Read the model definition and answer for the solid it produces. Units are mm, in the model's axes. A direction names the side the tool comes from. Give positions to 0.01 mm unless a question says otherwise; leave off trailing zeros. Write each loop counter-clockwise with the first axis right and the second up, starting at its lowest first coordinate (ties: lowest second). Pieces come first, ordered by that corner, then holes. Notation, with made-up numbers: M -27.5,61.5 L -11.5,61.5 A25 cw -11.5,88.5 Z; hole C 56.5,35.25 d11. An arc over 180 degrees is marked long. Use a Markdown table: item, result. Add a question column.
Item 1: The mould has two halves that part along Y. Classify faces 1 (the flat face through (15, -1, 3)), 2 (the cylindrical face through (-12.2, -1.8, -2.4)), 3 (the cylindrical face through (-9.06, 5.16, -4.73)): pulls with the +Y half, pulls with the -Y half, needs draft (parallel to the pull), parting line crosses it, or undercut.
Item 2: A cutting plane is placed at D-D on x = 12.25. Determine the outline of the cut face in (y, z).
Item 3: A cutting plane is placed at A-A on y = 0. Determine the outline of the cut face in (x, z) (3 decimals).
Item 4: Consider probe 1 along Y at (x, z) = (0, 13.85); probe 2 along X at (y, z) = (2.75, -0.25) (3 decimals); probe 3 along Y at (x, z) = (1.75, 10.25). Determine where each line is inside the solid, lowest interval first. Write a range as [from, to].
Item 5: Given P1, Ø3, axis at x = -8, y = -1.5, coming from the -Z side; P2, Ø3.5, axis at x = 0, y = 0, coming from the +Z side (3 decimals); P3, Ø5, axis at y = -3, z = 10.5, coming from the +X side; P4, Ø1.5, axis at x = -7.5, z = -2.5, coming from the -Y side, each flat-ended and moving along its own axis, determine where each tip first touches the part or whether it passes through.
Item 6: A cutting plane is placed at B-B on x = 1. Determine the outline of the cut face in (y, z) (3 decimals).
Item 7: For faces 4 (the cylindrical face through (-7, 0, -9)), 5 (the cylindrical face through (12, 0, 3)), 6 (the cylindrical face through (-3, 0, 12)), determine the directions among +Z, -Z, +X, -X, +Y, -Y from which every point of the face is accessible in a straight line to the end or side of a thin tool.
Item 8: A cutting plane is placed at C-C on z = -6.5. Determine the outline of the cut face in (x, y), then the cut area to 3 significant figures.
from build123d import *

# Parameters (mm, degrees)
SKETCH1_R           = 7
BOSS_EXTRUDE1_DEPTH = 15
SKETCH4_R           = 7
BOSS_EXTRUDE2_DEPTH = 15
SKETCH3_R           = 3
CUT_EXTRUDE1_DEPTH  = 5.625
CIRPATTERN1_COUNT   = 4


with BuildPart() as part:
    # Sketch1 → Boss-Extrude1 (new, symmetric)
    with BuildSketch(Plane.XY):
        Circle(SKETCH1_R)
    extrude(amount=BOSS_EXTRUDE1_DEPTH, both=True)

    # Sketch4 → Boss-Extrude2 (add, symmetric)
    with BuildSketch(Plane(origin=(0, 0, 0), x_dir=(0, 0, -1), z_dir=(1, 0, 0))):
        with Locations(Location((0, 0, 0), (0, 0, 270))):
            Circle(SKETCH4_R)
    extrude(amount=BOSS_EXTRUDE2_DEPTH, both=True)

    # Sketch3 → Cut-Extrude1 (cut)
    with BuildSketch(Plane.XY.offset(15)):
        Circle(SKETCH3_R)
    cut_extrude1 = extrude(amount=-CUT_EXTRUDE1_DEPTH, mode=Mode.SUBTRACT)

    # CirPattern1: Cut-Extrude1 ×4 about axis
    cirpattern1_axis = Axis((0, 0, 0), (0, 1, 0))
    for i in range(1, CIRPATTERN1_COUNT):
        add(cut_extrude1.rotate(cirpattern1_axis, i * 360 / CIRPATTERN1_COUNT), mode=Mode.SUBTRACT)


solid = part.part
Filled in:
| question | item | result |
|---|---|---|
| 1 | face 1 | needs draft |
| 1 | face 2 | undercut |
| 1 | face 3 | parting line crosses it |
| 2 | outline | C 0,0 d14; hole C 0,0 d6 |
| 3 | outline | M -15,-7 L -7,-7 L -7,-15 L -3,-15 L -3,-9.375 L 3,-9.375 L 3,-15 L 7,-15 L 7,-7 L 15,-7 L 15,-3 L 9.375,-3 L 9.375,3 L 15,3 L 15,7 L 7,7 L 7,15 L 3,15 L 3,9.375 L -3,9.375 L -3,15 L -7,15 L -7,7 L -15,7 L -15,3 L -9.375,3 L -9.375,-3 L -15,-3 Z |
| 4 | probe 1 | [-7, -3], [3, 7] |
| 4 | probe 2 | [-9.375, 9.375] |
| 4 | probe 3 | [-6.78, -2.44], [2.44, 6.78] |
| 5 | P1 | z = -15 |
| 5 | P2 | z = 9.375 |
| 5 | P3 | x = 6.98 |
| 5 | P4 | y = -6.78 |
| 6 | outline | M -6.928,-15 L -2.828,-15 L -2.828,-9.375 L 2.828,-9.375 L 2.828,-15 L 6.928,-15 L 6.928,-1 A7 ccw 6.928,1 L 6.928,15 L 2.828,15 L 2.828,9.375 L -2.828,9.375 L -2.828,15 L -6.928,15 L -6.928,1 A7 ccw -6.928,-1 Z |
| 7 | face 4 | -Z |
| 7 | face 5 | +X |
| 7 | face 6 | +Z |
| 8 | outline | M -15,-2.6 L -6.5,-2.6 A7 ccw 6.5,-2.6 L 15,-2.6 L 15,2.6 L 6.5,2.6 A7 ccw -6.5,2.6 L -15,2.6 Z |
| 8 | area | 239 mm² |
